Could you check a few things on this model? Use its own coordinates, in mm. A direction names the side the tool comes from. Round coordinates to 2 decimals unless told otherwise and drop trailing zeros. Write each loop counter-clockwise with the first axis right and the second up, starting at its lowest first coordinate (ties: lowest second). Pieces come first, ordered by that corner, then holes. Notation, with made-up numbers: (20, -39.75) -> (51, -39.75) arc R18 ccw to (51, -11.75) -> close; hole circle Ø2 at (63.5, 47.25). An arc over 180 degrees is marked (long way). One line per question, with ' | ' between items. Start each with the question number.
1. If I drill on line 1 along X through (y, z) = (-16, -93); line 2 along X through (y, z) = (-24, -82.5); line 3 along Z through (x, y) = (49, -15), over which ranges is the centre line in solid material (lowest first)? Write a range as [from, to].
2. Imagine slicing it at D-D, the plane z = 8. List the corners of the cut face in (x, y) for me, and give its area (3 significant figures).
3. For pin 1 Ø3 at (x, y) = (-57, -14) entering from +Z; pin 2 Ø1.5 at (x, y) = (7, -49) entering from -Z; pin 3 Ø3.5 at (x, z) = (-95, 0.5) entering from -Y, each with a flat end and sliding along its axis, tell me the tip position at first contact or that it passes through.
4. Imagine slicing it at C-C, the plane z = -54. List the corners of the cut face in (x, y) for me.
5. Thinking about a two-plate mould opening in Y: for faces 4 (the flat face through (-1, -25, 28)), 5 (the flat face through (-11.585, -23.313, -106.991)), 6 (the flat face through (-44, -23.085, -122)), which applies, released by +Y, released by -Y, zero draft, split by the parting line, or undercut?
6. For faces 1 (the flat face through (-51.788, -21, -116)), 2 (the flat face through (-98.4, -29, 1)), 3 (the flat face through (76.2, -24.4, -109.651)), which set-ups out of +Z, -Z, +X, -X, +Y, -Y let a thin tool reach every point of the face, with its end or its side?
7. Imagine slicing it at B-B, the plane x = 70. List the corners of the cut face in (y, z) for me, and give its area (3 significant figures).
8. Imagine slicing it at A-A, the plane x = 49. List the corners of the cut face in (y, z) for me.
from build123d import *

# Parameters (mm, degrees)
F0_W           = 200
F0_H           = 56
F1_DEPTH       = 50
F2_T           = -6
F3_W           = 149.0980237722
F3_H           = 8.3
F4_DEPTH       = 98.5
F4_DEPTH_BACK  = 98.4
F5_R           = 2.1479446761
F6_DEPTH       = 3.7
F7_W           = 200
F7_H           = 48.0854995549
F8_DEPTH       = 98.2
F9_W           = 44.6983203292
F9_H           = 8.100832057
F10_DEPTH      = 25
F11_W          = 43.396525085
F11_H          = 74.3940398097
F12_DEPTH      = 55.1
F12_DEPTH_BACK = 75
F13_W          = 24.1317078471
F13_H          = 25.4259835929
F14_DEPTH      = 29.4
F16_DEPTH      = 50.3
F17_W          = 57.2261828929
F17_H          = 32.9050645232
F18_DEPTH      = 25


# Not quite as in the source:
# - a pattern or mirror of a feature is missing from the dataset's text; its kind, count and spacing are read off the source's solid


with BuildPart() as f1:
    # F0 (on Front) → F1 (new body)
    with BuildSketch(Plane.XZ):
        Rectangle(F0_W, F0_H)
    extrude(amount=F1_DEPTH)

    # F2
    f2_openings = [f1.faces().sort_by_distance(p)[0] for p in [
        (0, -50, 0),
    ]]
    offset(amount=F2_T, openings=f2_openings)

    # F3 (on Right) → F4 (cut, two sides)
    with BuildSketch(Plane.YZ) as f4_sk:
        with Locations((-82.4490264058, 0.55)):
            Rectangle(F3_W, F3_H)
    extrude(amount=F4_DEPTH, mode=Mode.SUBTRACT)
    extrude(f4_sk.sketch, amount=-F4_DEPTH_BACK, mode=Mode.SUBTRACT)

    # F5 (on face) → F6 (join)
    with BuildSketch(Plane.XY.offset(28)):
        with Locations((-46.3078469038, -5.0663095899)):
            Circle(F5_R)
    extrude(amount=F6_DEPTH)

    # F7 (on face) → F8 (join)
    with BuildSketch(Plane(origin=(0, 0, -28), x_dir=(1, 0, 0), z_dir=(0, 0, -1))):
        with Locations((0, 24.0427497774)):
            Rectangle(F7_W, F7_H)
    extrude(amount=F8_DEPTH)

    # F9 (on face) → F10 (cut)
    with BuildSketch(Plane.XZ.offset(48.0854995549)):
        with Locations((-59.1169446707, -122.1495839715)):
            Rectangle(F9_W, F9_H)
    f10 = extrude(amount=-F10_DEPTH, mode=Mode.SUBTRACT)

    # F10_copies: F10 across plane
    add(f10.mirror(Plane(origin=(0, 0, 0), x_dir=(0, 0, 1), z_dir=(1, 0, 0))), mode=Mode.SUBTRACT)

    # F11 (on Front) → F12 (cut, two sides)
    with BuildSketch(Plane.XZ) as f12_sk:
        with Locations((-61.3989308476, -72.4539384246)):
            Rectangle(F11_W, F11_H)
    f12 = extrude(amount=-F12_DEPTH, mode=Mode.SUBTRACT) + extrude(f12_sk.sketch, amount=F12_DEPTH_BACK, mode=Mode.SUBTRACT)

    # F12_copies: F12 across plane
    add(f12.mirror(Plane(origin=(0, 0, 0), x_dir=(0, 0, 1), z_dir=(1, 0, 0))), mode=Mode.SUBTRACT)

    # F13 (on face) → F14 (cut)
    with BuildSketch(Plane.XY.offset(-109.6509583294)):
        with Locations((-63.8535097241, -23.7910989672)):
            Rectangle(F13_W, F13_H)
    f14 = extrude(amount=-F14_DEPTH, mode=Mode.SUBTRACT)

    # F14_copies: F14 across plane
    add(f14.mirror(Plane(origin=(0, 0, 0), x_dir=(0, 0, 1), z_dir=(1, 0, 0))), mode=Mode.SUBTRACT)

    # F15 (on face) → F16 (cut)
    with BuildSketch(Plane(origin=(0, 0, -126.2), x_dir=(1, 0, 0), z_dir=(0, 0, -1))):
        Polygon((16.0494638515, 30.4643716825), (8.6599005478, 44.7303298699), (-7.3895633037, 45.4637594198), (-16.0494638515, 31.9312307822), (-8.6599005478, 17.6652725948), (7.3895633037, 16.9318430449), align=None)
    extrude(amount=-F16_DEPTH, mode=Mode.SUBTRACT)

    # F17 (on face) → F18 (cut)
    with BuildSketch(Plane.XZ.offset(48.0854995549)):
        with Locations((4.1727414355, -87.4758176506)):
            Rectangle(F17_W, F17_H)
    extrude(amount=-F18_DEPTH, mode=Mode.SUBTRACT)


solid = f1.part
Geometry results:
1) line 1: x = [-100, -83.1], [-39.7, 39.7], [83.1, 100] | line 2: x = [-100, -83.1], [-39.7, -24.44], [32.79, 39.7], [83.1, 100] | line 3: z = [-126.2, -109.65], [-35.26, -22], [22, 28]
2) outline: (-100, -50) -> (-94, -50) -> (-94, -6) -> (94, -6) -> (94, -50) -> (100, -50) -> (100, 0) -> (-100, 0) -> close | area: 1,730 mm2
3) pin 1: stops at z = 28 | pin 2: stops at z = -28 | pin 3: stops at y = -7.9
4) outline: (-100, -48.09) -> (-83.1, -48.09) -> (-83.1, 0) -> (-100, 0) -> close; (-39.7, -48.09) -> (39.7, -48.09) -> (39.7, 0) -> (-39.7, 0) -> close; (83.1, -48.09) -> (100, -48.09) -> (100, 0) -> (83.1, 0) -> close
5) face 4: zero draft | face 5: undercut | face 6: released by -Y
6) face 1: -Z | face 2: -Y | face 3: +Y, -Y
7) outline: (-50, -28) -> (-48.09, -28) -> (-48.09, -35.26) -> (0, -35.26) -> (0, 28) -> (-50, 28) -> (-50, 22) -> (-6, 22) -> (-6, -22) -> (-50, -22) -> close; (-48.09, -118.1) -> (-36.5, -118.1) -> (-36.5, -109.65) -> (-48.09, -109.65) -> close; (-11.08, -126.2) -> (0, -126.2) -> (0, -109.65) -> (-11.08, -109.65) -> close | area: 1,490 mm2
8) outline: (-50, -28) -> (-48.09, -28) -> (-48.09, -35.26) -> (0, -35.26) -> (0, 28) -> (-50, 28) -> (-50, 22) -> (-6, 22) -> (-6, -22) -> (-50, -22) -> close; (-48.09, -118.1) -> (-23.09, -118.1) -> (-23.09, -126.2) -> (0, -126.2) -> (0, -109.65) -> (-48.09, -109.65) -> close
